Check sheet for the modelled part. Datum: model origin and axes. Units: mm. A direction names the side the tool comes from. Round coordinates to 2 decimals unless told otherwise and drop trailing zeros. One line per item, written item: value.
from build123d import *
from build123d.topology import SkipClean

# Parameters (mm, degrees)
BASE_FLANGE1_DEPTH                           = 14
CBORE_FOR_M8_HEX_SOCKET_HEAD_CAP_SCR_2_COUNT = 2
CBORE_FOR_M8_HEX_SOCKET_HEAD_CAP_SCR_2_PITCH = 30
M4_TAPPED_HOLE1_AT_2_COUNT                   = 2
M4_TAPPED_HOLE1_AT_2_PITCH                   = 31.112698372
M4_TAPPED_HOLE1_AT_3_COUNT                   = 2
M4_TAPPED_HOLE1_AT_3_PITCH                   = 44
M4_TAPPED_HOLE1_AT_4_COUNT                   = 2
M4_TAPPED_HOLE1_AT_4_PITCH                   = 31.112698372
CIRPATTERN1_COUNT                            = 4
FILLET2_R                                    = 6
FILLET1_R                                    = 2
CHAMFER1_SIZE                                = 0.8
CHAMFER2_SIZE                                = 0.8


# Sheet-metal steps are written as plain solids
with BuildPart() as part:
    # Sketch1 → Base-Flange1 (new body)
    with BuildSketch(Plane.XY):
        with BuildLine():
            Line((0, 0), (-65, 0))
            Line((-65, 0), (-65, 60))
            Line((-65, 60), (-32.5, 78.763883749))
            Line((-32.5, 78.763883749), (-32.5, 102.5))
            Line((-32.5, 102.5), (0, 102.5))
            Line((0, 102.5), (0, 88))
            ThreePointArc((0, 88), (-18, 70), (0, 52))
            Line((0, 52), (0, 0))
        make_face()
    extrude(amount=-BASE_FLANGE1_DEPTH)

    # Sketch7 → CBORE for M8 Hex Socket Head Cap Screw1 (revolve, cut)
    with BuildSketch(Plane(origin=(-50, 45, 0), x_dir=(0, -1, 0), z_dir=(1, 0, 0))):
        Polygon((0, 0), (0, 14), (4.525, 14), (4.25, 13.725), (4.25, 8.6), (7, 8.6), (7, 0.525), (7.525, 0), align=None)
    cbore_for_m8_hex_socket_head_cap_screw1 = revolve(axis=Axis((-50, 45, 6.35), (0, 0, -1)), mode=Mode.SUBTRACT)

    # CBORE for M8 Hex Socket Head Cap Scr 2: CBORE for M8 Hex Socket Head Cap Screw1 ×2
    with Locations(*[(0, -i * CBORE_FOR_M8_HEX_SOCKET_HEAD_CAP_SCR_2_PITCH, 0) for i in range(1, CBORE_FOR_M8_HEX_SOCKET_HEAD_CAP_SCR_2_COUNT)]):
        add(cbore_for_m8_hex_socket_head_cap_screw1, mode=Mode.SUBTRACT)

    # Sketch18 → CBORE for M6 Hex Socket Head Cap Screw1 (revolve, cut)
    with BuildSketch(Plane(origin=(-20, 15, 0), x_dir=(0, -1, 0), z_dir=(1, 0, 0))):
        Polygon((0, 0), (0, 14), (3.5, 14), (3.25, 13.75), (3.25, 6.5), (5.5, 6.5), (5.5, 0.25), (5.75, 0), align=None)
    revolve(axis=Axis((-20, 15, 6.35), (0, 0, -1)), mode=Mode.SUBTRACT)

    # Mirror1: part across plane


with BuildPart() as part_1:
    with SkipClean():  # the faces are left unmerged after this step: merging them gives an invalid solid
        add(part.part)
        add(part.part.mirror(Plane(origin=(0, 102.5, -14), x_dir=(0, 0, 1), z_dir=(1, 0, 0))))

    # Sketch12 → M4 Tapped Hole1 (revolve, cut)
    with SkipClean():  # the faces are left unmerged after this step: merging them gives an invalid solid
        with BuildSketch(Plane(origin=(-22, 70, 0), x_dir=(0, -1, 0), z_dir=(1, 0, 0))):
            Polygon((0, 0), (0, 14), (2, 14), (1.65, 13.65), (1.65, 0.35), (2, 0), align=None)
        m4_tapped_hole1 = revolve(axis=Axis((-22, 70, 6.35), (0, 0, -1)), mode=Mode.SUBTRACT)

    # M4 Tapped Hole1 at 2: M4 Tapped Hole1 ×2
    with SkipClean():  # the faces are left unmerged after this step: merging them gives an invalid solid
        with Locations(*[Vector(0.7071067811865477, 0.7071067811865474, 0) * (i * M4_TAPPED_HOLE1_AT_2_PITCH) for i in range(1, M4_TAPPED_HOLE1_AT_2_COUNT)]):
            add(m4_tapped_hole1, mode=Mode.SUBTRACT)

    # M4 Tapped Hole1 at 3: M4 Tapped Hole1 ×2
    with SkipClean():  # the faces are left unmerged after this step: merging them gives an invalid solid
        with Locations(*[(i * M4_TAPPED_HOLE1_AT_3_PITCH, 0, 0) for i in range(1, M4_TAPPED_HOLE1_AT_3_COUNT)]):
            add(m4_tapped_hole1, mode=Mode.SUBTRACT)

    # M4 Tapped Hole1 at 4: M4 Tapped Hole1 ×2
    with SkipClean():  # the faces are left unmerged after this step: merging them gives an invalid solid
        with Locations(*[Vector(0.7071067811865475, -0.7071067811865477, 0) * (i * M4_TAPPED_HOLE1_AT_4_PITCH) for i in range(1, M4_TAPPED_HOLE1_AT_4_COUNT)]):
            add(m4_tapped_hole1, mode=Mode.SUBTRACT)

    # Sketch15 → CBORE for M5 Hex Socket Head Cap Screw1 (revolve, cut)
    with SkipClean():  # the faces are left unmerged after this step: merging them gives an invalid solid
        with BuildSketch(Plane(origin=(23.550191347, 93.550191347, -14), x_dir=(0, 1, 0), z_dir=(1, 0, 0))):
            Polygon((0, 0), (0, 14), (3, 14), (2.75, 13.75), (2.75, 5.5), (4.75, 5.5), (4.75, 0.5), (5.25, 0), align=None)
        cbore_for_m5_hex_socket_head_cap_screw1 = revolve(axis=Axis((23.550191347, 93.550191347, -20.35), (0, 0, 1)), mode=Mode.SUBTRACT)

    # CirPattern1: CBORE for M5 Hex Socket Head Cap Screw1 ×4 about axis
    with SkipClean():  # the faces are left unmerged after this step: merging them gives an invalid solid
        cirpattern1_axis = Axis((0, 70, 0), (0, 0, 1))
        for i in range(1, CIRPATTERN1_COUNT):
            add(cbore_for_m5_hex_socket_head_cap_screw1.rotate(cirpattern1_axis, i * 360 / CIRPATTERN1_COUNT), mode=Mode.SUBTRACT)

    # Fillet2
    fillet2_edges = [part_1.edges().sort_by_distance(p)[0] for p in [
        (-32.5, 78.763883749, -7),
        (32.5, 78.763883749, -7),
    ]]
    fillet(fillet2_edges, radius=FILLET2_R)

    # Fillet1
    fillet1_edges = [part_1.edges().sort_by_distance(p)[0] for p in [
        (-65, 60, -7),
        (-32.5, 102.5, -7),
        (-65, 0, -7),
        (65, 60, -7),
        (32.5, 102.5, -7),
        (65, 0, -7),
    ]]
    fillet(fillet1_edges, radius=FILLET1_R)

    # Chamfer1
    chamfer1_edges = [part_1.edges().sort_by_distance(p)[0] for p in [
        (49.75, 68.804591605, 0),
        (49.75, 68.804591605, -14),
        (-49.75, 68.804591605, 0),
        (-49.75, 68.804591605, -14),
        (33.303847577, 79.227985364, 0),
        (33.303847577, 79.227985364, -14),
        (-33.303847577, 79.227985364, 0),
        (-33.303847577, 79.227985364, -14),
        (-31.5, 0, 0),
        (-31.5, 0, -14),
        (32.5, 91.363992682, 0),
        (-15.25, 102.5, 0),
        (-32.5, 91.363992682, 0),
        (-65, 30.422649731, 0),
        (65, 30.422649731, 0),
        (-64.732050808, 59.845299462, 0),
        (-31.914213562, 101.914213562, 0),
        (31.914213562, 101.914213562, 0),
        (64.732050808, 59.845299462, 0),
        (-64.414213562, 0.585786438, 0),
        (64.414213562, 0.585786438, 0),
        (65, 30.422649731, -14),
        (-15.25, 102.5, -14),
        (32.5, 91.363992682, -14),
        (-65, 30.422649731, -14),
        (-32.5, 91.363992682, -14),
        (-64.732050808, 59.845299462, -14),
        (-31.914213562, 101.914213562, -14),
        (31.914213562, 101.914213562, -14),
        (64.732050808, 59.845299462, -14),
        (-64.414213562, 0.585786438, -14),
        (64.414213562, 0.585786438, -14),
    ]]
    chamfer(chamfer1_edges, length=CHAMFER1_SIZE)

    # Chamfer2
    chamfer2_edges = [part_1.edges().sort_by_distance(p)[0] for p in [
        (-18, 70, 0),
        (-18, 70, -14),
    ]]
    chamfer(chamfer2_edges, length=CHAMFER2_SIZE)


solid = part_1.part
Item 1: Sectioned sample at A-A on x = -50. Count the separate pieces of the cut face and the enclosed holes in it, and give its area (3 significant figures).
Answer:
separate pieces: 3
enclosed holes: 0
area: 627 mm^2
Item 2: Thickness scan on line 1 (X direction, y = 15, z = -10.2); line 2 (Y direction, x = 55, z = -4.75); line 3 (X direction, y = 97, z = -12). Record the ranges inside material, lowest first.
Answer:
line 1: x = -65 to -54.25, -45.75 to -23.25, -16.75 to 16.75, 23.25 to 45.75, 54.25 to 65
line 2: y = 0 to 10.1, 19.9 to 40.1, 49.9 to 65.77
line 3: x = -32.5 to -26.82, -20.29 to 20.29, 26.82 to 32.5
Item 3: Tool access check on faces 1 (the cylindrical face through (-22.72, 43.83, -4.43)), 2 (the flat face through (-50, 20, -8.6)). Record the directions out of +Z, -Z, +X, -X, +Y, -Y that give a thin tool (end or side, any length) a straight path to the whole face; none if there is none.
Answer:
face 1: +Z, -Z
face 2: +Z
Item 4: Mould release check, pull along X, two halves, no side actions. Record for faces 3 (the flat face through (49.747, 68.338, -13.606)), 4 (the flat face through (-45, 45, -8.6)): pulls with the +X half, pulls with the -X half, needs draft (parallel to the pull), parting line crosses it, or undercut.
Answer:
face 3: pulls with the +X half
face 4: undercut
Item 5: Depth check by flat-ended pin: P1, Ø3.5, axis at x = -18, y = 13.5, coming from the +Z side; P2, Ø6.5, axis at x = 23.55, y = 46.45, coming from the -Z side; P3, Ø8, axis at y = 80, z = -5, coming from the -X side. Enter the tip coordinate at first touch or a pass-through.
Answer:
P1: stops at z = -6.5
P2: stops at z = -8.5
P3: stops at x = -37.29
